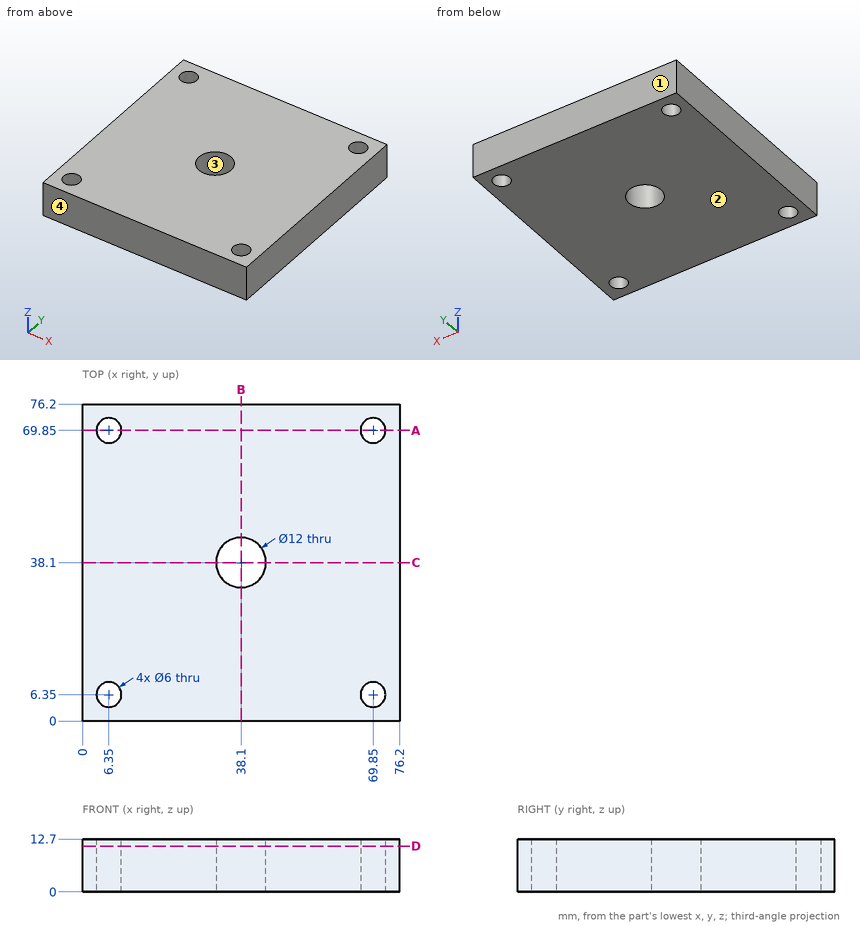
Here's the drawing with two shaded views (mm, measured from the low corner). I have some questions. Give positions to 0.01 mm unless a question says otherwise; leave off trailing zeros. Loops run counter-clockwise (first coordinate to the right, second up) from the corner with the lowest first, then second, coordinate; pieces in that order, holes last. Notation, with made-up numbers: (-27.75, 66) -> (0.25, 66) arc R32 cw to (0.25, 101) -> close; hole circle Ø6 at (56, 38). An arc over 180 degrees is marked (long way). Answer as a JSON object with one key per item and string values. Group by question number.
Item 1: Imagine slicing it at A-A on y = 69.85. Write out the boundary of the cut face in (x, z), then the cut area to 3 significant figures.
Item 2: Imagine slicing it at B-B on x = 38.1. Write out the boundary of the cut face in (y, z).
Item 3: I need wall thicknesses on L1, parallel to Y at x = 6.35, z = 6.25; L2, parallel to Y at x = 69, z = 10.25; L3, parallel to X at y = 36, z = 7. Which ranges of each line are inside material? Lowest first, please.
Item 4: Imagine slicing it at D-D on z = 11. Write out the boundary of the cut face in (x, y), then the cut area to 3 significant figures.
Item 5: Thinking about a two-plate mould opening in Y: for the marked faces 1, 2, 3 and 4, which applies, pulls with the +Y half, pulls with the -Y half, needs draft (parallel to the pull), parting line crosses it, or undercut?
Answer list:
{
 "1": {"outline": "(0, 0) -> (3.35, 0) -> (3.35, 12.7) -> (0, 12.7) -> close; (9.35, 0) -> (66.85, 0) -> (66.85, 12.7) -> (9.35, 12.7) -> close; (72.85, 0) -> (76.2, 0) -> (76.2, 12.7) -> (72.85, 12.7) -> close", "area": "815 mm2"},
 "2": {"outline": "(0, 0) -> (32.1, 0) -> (32.1, 12.7) -> (0, 12.7) -> close; (44.1, 0) -> (76.2, 0) -> (76.2, 12.7) -> (44.1, 12.7) -> close"},
 "3": {"L1": "y = 0 to 3.35, 9.35 to 66.85, 72.85 to 76.2", "L2": "y = 0 to 3.47, 9.23 to 66.97, 72.73 to 76.2", "L3": "x = 0 to 32.48, 43.72 to 76.2"},
 "4": {"outline": "(0, 0) -> (76.2, 0) -> (76.2, 76.2) -> (0, 76.2) -> close; hole circle Ø6 at (6.35, 6.35); hole circle Ø6 at (6.35, 69.85); hole circle Ø12 at (38.1, 38.1); hole circle Ø6 at (69.85, 6.35); hole circle Ø6 at (69.85, 69.85)", "area": "5,580 mm2"},
 "5": {"face 1": "pulls with the +Y half", "face 2": "needs draft", "face 3": "undercut", "face 4": "pulls with the -Y half"}
}
